Source: CAD feature listing. Evaluate the final solid. Frame: model axes, mm. A direction names the side the tool comes from. Coordinates: 2 decimals unless noted, no trailing zeros. Loops run counter-clockwise (first coordinate to the right, second up) from the corner with the lowest first, then second, coordinate; pieces in that order, holes last.
```python
from build123d import *

# Parameters (mm, degrees)
OUTLET_SOCKET_SKETCH_W = 15
OUTLET_SOCKET_SKETCH_H = 10


with BuildPart() as part:
    # Regulator_Ninja Sketch → Regulator_Ninja (revolve)
    with BuildSketch(Plane.XY, mode=Mode.PRIVATE) as regulator_ninja_sk:
        Polygon((14, 0), (14, 7.2), (0, 7.2), (0, 19), (-65, 19), (-65, 0), align=None)
    revolve(regulator_ninja_sk.sketch.rotate(Axis((-1000, 0, 0), (1, 0, 0)), 90), axis=Axis((-1000, 0, 0), (1, 0, 0)))

    # Outlet Socket Sketch → Outlet Socket (revolve, cut)
    with BuildSketch(Plane.XY, mode=Mode.PRIVATE) as outlet_socket_sk:
        with Locations((-58.5, 5)):
            Rectangle(OUTLET_SOCKET_SKETCH_W, OUTLET_SOCKET_SKETCH_H)
    revolve(outlet_socket_sk.sketch.rotate(Axis((-1000, 0, 0), (1, 0, 0)), 90), axis=Axis((-1000, 0, 0), (1, 0, 0)), mode=Mode.SUBTRACT)


solid = part.part
```
Q1. Draft query along Y for faces 3 (the flat face through (14, 0, 0)), 4 (the cylindrical face through (-58, 0, -10)), 5 (the cylindrical face through (6.9, -2.16, 6.87)), 6 (the flat face through (-51, 0, 0)). Return one class per face: released by +Y, released by -Y, zero draft, split by the parting line, or undercut.
Q2. Section query D-D on y = -8.5. Return the cut outline in (x, z).
Q3. Material intervals for line 1 along Y through (x, z) = (-55.75, 0); line 2 along X through (y, z) = (0, -3); line 3 along X through (y, z) = (-8.5, -6.5), sorted ascending.
Q4. Section query A-A on z = 0. Return the cut outline in (x, y), then the cut area to 3 significant figures.
Q5. First-contact query: pin 1 Ø6 at (x, y) = (-13.5, -8) entering from +Z; pin 2 Ø1 at (x, y) = (-29, 13) entering from +Z; pin 3 Ø6 at (y, z) = (1, 2) entering from -X; pin 4 Ø6 at (y, z) = (-4.5, -8.5) entering from +X. Flat tips, straight axial feed; report the tip coordinate or a pass-through.
Q6. Section query C-C on x = -35. Return the cut outline in (y, z).
Q7. Reachability of faces 1 (the flat face through (0, 0, -8)), 2 (the flat face through (-65, 8, 8)) from +Z, -Z, +X, -X, +Y, -Y: full face, straight path, thin tool, end or side. Return the list, or none.
Resolved:
1. face 3: zero draft
1. face 4: undercut
1. face 5: split by the parting line
1. face 6: undercut
2. outline: (-65, -16.99) - (0, -16.99) - (0, 16.99) - (-65, 16.99) - (-65, 5.27) - (-51, 5.27) - (-51, -5.27) - (-65, -5.27) - close
3. line 1: y = -19 to -10, 10 to 19
3. line 2: x = -51 to 14
3. line 3: x = -65 to 0
4. outline: (-65, -19) - (0, -19) - (0, -7.2) - (14, -7.2) - (14, 7.2) - (0, 7.2) - (0, 19) - (-65, 19) - (-65, 10) - (-51, 10) - (-51, -10) - (-65, -10) - close
4. area: 2,390 mm2
5. pin 1: stops at z = 18.33
5. pin 2: stops at z = 14.31
5. pin 3: stops at x = -51
5. pin 4: stops at x = 14
6. outline: circle Ø38 at (0, 0)
7. face 1: +X
7. face 2: +Z, -Z, -X, +Y, -Y
